```python
from build123d import *

# Parameters (mm, degrees)
EXTRUDE_1_DEPTH     = 15
SKETCH_3_R          = 1.75
CUT_EXTRUDE_2_DEPTH = 55.598534779
EXTRUDE_2_DEPTH     = 10
EXTRUDE_START       = -5
EXTRUDE_3_DEPTH     = 5
CUT_EXTRUDE_5_REACH = 60.097
SKETCH_6_R          = 2.75
SKETCH_7_R          = 5
CUT_EXTRUDE_6_DEPTH = 5
SKETCH_10_W         = 6
SKETCH_10_H         = 6
CUT_EXTRUDE_7_DEPTH = 2
SKETCH_11_W         = 6
SKETCH_11_H         = 6
CUT_EXTRUDE_8_DEPTH = 2


with BuildPart() as part:
    # 草图1 → 凸台-拉伸1 (new body)
    with BuildSketch(Plane.XY):
        Polygon((0, 0), (0, 16), (6, 16), (6, 5), (44, 5), (44, 16), (50, 16), (50, 0), align=None)
    extrude(amount=EXTRUDE_1_DEPTH)

    # 草图3 → 切除-拉伸2 (cut, through all)
    with BuildSketch(Plane(origin=(50, 0, 0), x_dir=(0, 0, -1), z_dir=(1, 0, 0))):
        with Locations(Location((-7.5, 8.5, 0), (0, 0, 90))):
            Circle(SKETCH_3_R)
        with BuildLine():
            Line((-14.5, 8.5), (-23.066471686, 8.5))
            Line((-23.066471686, 8.5), (-23.066471686, 64.301280236))
            Line((-23.066471686, 64.301280236), (5.906378089, 64.301280236))
            Line((5.906378089, 64.301280236), (5.906378089, 8.5))
            Line((5.906378089, 8.5), (-0.5, 8.5))
            ThreePointArc((-0.5, 8.5), (-7.5, 15.5), (-14.5, 8.5))
        make_face()
    extrude(amount=-CUT_EXTRUDE_2_DEPTH, mode=Mode.SUBTRACT)

    # 草图8 → 凸台-拉伸2 (add)
    with BuildSketch(Plane.XZ):
        with BuildLine():
            Line((15, 15), (21, 15))
            ThreePointArc((21, 15), (16.5, 7.5), (21, 0))
            Line((21, 0), (15, 0))
            ThreePointArc((15, 0), (12.5, 7.5), (15, 15))
        make_face()
        with BuildLine():
            Line((29, 15), (35, 15))
            ThreePointArc((35, 15), (37.5, 7.5), (35, 0))
            Line((35, 0), (29, 0))
            ThreePointArc((29, 0), (33.5, 7.5), (29, 15))
        make_face()
    extrude(amount=EXTRUDE_2_DEPTH)

    # 草图9 → 凸台-拉伸3 (add)
    with BuildSketch(Plane.XZ.offset(10).offset(EXTRUDE_START)):
        with BuildLine():
            Line((21, 15), (29, 15))
            Line((29, 15), (35, 15))
            ThreePointArc((35, 15), (37.5, 7.5), (35, 0))
            Line((35, 0), (29, 0))
            Line((29, 0), (21, 0))
            Line((21, 0), (15, 0))
            ThreePointArc((15, 0), (12.5, 7.5), (15, 15))
            Line((15, 15), (21, 15))
        make_face()
    extrude(amount=EXTRUDE_3_DEPTH)

    # 切除-拉伸5: up to this face of the body (flat: up to its plane)
    cut_extrude_5_end = Plane(part.part.faces().sort_by_distance((25, 5, 7.5))[0])
    # 草图6 → 切除-拉伸5 (cut, up to the picked face)
    with BuildSketch(Plane.XZ.offset(10), mode=Mode.PRIVATE) as cut_extrude_5_sk1:
        with Locations((25, 7.5)):
            Circle(SKETCH_6_R)
    cut_extrude_5_tool1 = split(extrude(cut_extrude_5_sk1.sketch, amount=-CUT_EXTRUDE_5_REACH, mode=Mode.PRIVATE), bisect_by=cut_extrude_5_end, keep=Keep.BOTH, mode=Mode.PRIVATE)
    add(cut_extrude_5_tool1.solids().sort_by(Axis((25, -10, 7.5), (0, 1, 0)))[0], mode=Mode.SUBTRACT)

    # 草图7 → 切除-拉伸6 (cut)
    with BuildSketch(Plane(origin=(0, 5, 0), x_dir=(1, 0, 0), z_dir=(0, 1, 0))):
        with Locations(Location((25, -7.5, 0), (0, 0, 180))):
            Circle(SKETCH_7_R)
    extrude(amount=-CUT_EXTRUDE_6_DEPTH, mode=Mode.SUBTRACT)

    # 草图10 → 切除-拉伸7 (cut)
    with BuildSketch(Plane.ZY.offset(-44)):
        with Locations((7.5, 8.5)):
            Rectangle(SKETCH_10_W, SKETCH_10_H)
    extrude(amount=-CUT_EXTRUDE_7_DEPTH, mode=Mode.SUBTRACT)

    # 草图11 → 切除-拉伸8 (cut)
    with BuildSketch(Plane(origin=(6, 0, 0), x_dir=(0, 0, -1), z_dir=(1, 0, 0))):
        with Locations((-7.5, 8.5)):
            Rectangle(SKETCH_11_W, SKETCH_11_H)
    extrude(amount=-CUT_EXTRUDE_8_DEPTH, mode=Mode.SUBTRACT)


solid = part.part
```
Verification items for the finished model (mm, model axes). A direction names the side the tool comes from. Give positions to 0.01 mm unless a question says otherwise; leave off trailing zeros. Loops run counter-clockwise (first coordinate to the right, second up) from the corner with the lowest first, then second, coordinate; pieces in that order, holes last. Notation, with made-up numbers: M 68,-9 L 118,-9 A23 cw 118,16 Z; hole C 75.25,50 d3. An arc over 180 degrees is marked long. Return JSON: item names as keys, results as strings.
1) Section check D-D, the plane y = 3. Enter the section's corners in (x, z).
Findings:
{"outline": "M 0,0 L 50,0 L 50,15 L 0,15 Z; hole C 25,7.5 d10"}
2) Section check C-C, the plane x = 25. Enter the section's corners in (y, z).
Findings:
{"outline": "M -10,0 L -5,0 L -5,4.75 L -10,4.75 Z; M -10,10.25 L -5,10.25 L -5,15 L -10,15 Z; M 0,0 L 5,0 L 5,2.5 L 0,2.5 Z; M 0,12.5 L 5,12.5 L 5,15 L 0,15 Z"}
3) Gauge pin test, flat ends, axial feed: P1, Ø1, axis at x = 45, y = 9.5, coming from the +Z side; P2, Ø1.8, axis at y = 8.5, z = 7.5, coming from the -X side; P3, Ø8, axis at y = -6.5, z = 4, coming from the -X side; P4, Ø3, axis at x = 44, z = 11, coming from the +Y side. Record the tip position at first contact, or that the pin passes through.
Findings:
{"P1": "stops at z = 14.48", "P2": "passes through", "P3": "stops at x = 12.5", "P4": "stops at y = 15.21"}
4) Section check A-A, the plane x = 5.5. Enter the section's corners in (y, z).
Findings:
{"outline": "M 0,0 L 8.5,0 L 8.5,0.5 A7 ccw 8.5,14.5 L 8.5,15 L 0,15 Z; hole M 5.5,4.5 L 11.5,4.5 L 11.5,10.5 L 5.5,10.5 Z"}
5) Section check B-B, the plane y = -3. Enter the section's corners in (x, z).
Findings:
{"outline": "M 15,0 L 21,0 A8.5 cw 21,15 L 15,15 A12.5 ccw Z; M 29,0 L 35,0 A12.5 ccw 35,15 L 29,15 A8.5 cw Z"}
6) Material ranges on L1, parallel to X at y = 5.75, z = 10.25; L2, parallel to X at y = 13, z = 6.75; L3, parallel to Y at x = 30.5, z = 1.25, recorded low to high. Write a range as [from, to].
Findings:
{"L1": "x = [0, 4], [46, 50]", "L2": "x = [0, 6], [44, 50]", "L3": "y = [-10, -5], [0, 5]"}
7) Tool access check on faces 1 (the cylindrical face through (3.04, 15.5, 7.35)), 2 (the cylindrical face through (29.995, 2.535, 7.72)), 3 (the flat face through (25, 1, 15)), 4 (the flat face through (6, 13, 7)), 5 (the flat face through (45, 8, 10.5)). Record the directions out of +Z, -Z, +X, -X, +Y, -Y that give a thin tool (end or side, any length) a straight path to the whole face; none if there is none.
Findings:
{"face 1": "+X, -X, +Y", "face 2": "+Y", "face 3": "+Z, +X, -X, +Y, -Y", "face 4": "+Z, -Z, +Y", "face 5": "none"}
8) Mould release check, pull along X, two halves, no side actions. Record for faces 6 (the cylindrical face through (37.5, -4.9, 7.6)), 7 (the flat face through (44, 13, 7)), 8 (the flat face through (25, 1, 0)): released by +X, released by -X, zero draft, split by the parting line, or undercut.
Findings:
{"face 6": "released by +X", "face 7": "undercut", "face 8": "zero draft"}
